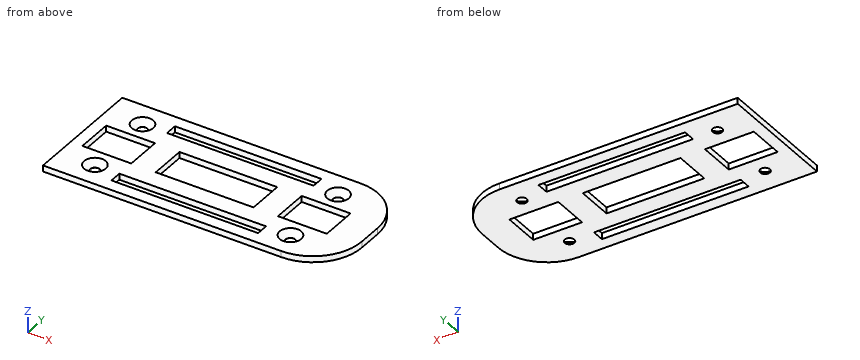
from build123d import *
from build123d import SkipClean  # not in build123d's __all__

# Parameters (mm, degrees)
F1_DEPTH        = 31.75
F1_DEPTH_BACK   = 31.75
F3_R            = 6.35
F4_DEPTH        = 149.1828857926
F5_R            = 12.7
F6_DEPTH        = 25.4
F7_R            = 9.525
F8_DEPTH        = 44.45
F8_DEPTH_BACK   = 66.9427915833
F10_D           = 4.2
F10_DEPTH       = 25.4
F10_TIP         = 1.2618073
F12_DEPTH       = 3.175
F14_D           = 5
F14_CSINK_D     = 11.2
F14_CSINK_ANGLE = 90
F15_W           = 25.4
F15_H           = 19.05
F15_W_2         = 76.2
F15_H_2         = 6.35
F15_W_3         = 50.8
F16_DEPTH       = 41.2760001


# Not quite as in the source:
# - a feature of the source that left no trace in its solid (it failed there, or was rolled back) is left out


with BuildPart() as f1:
    # F0 (on Front) → F1 (new body, two sides)
    with BuildSketch(Plane.XZ) as f1_sk:
        with BuildLine():
            Line((66.9417914833, 19.05), (-82.2400942093, 19.05))
            Line((-82.2400942093, 19.05), (-82.2400942093, -19.05))
            add(Edge.make_bspline(
                [(-82.2400942093, -19.05), (0, -19.05), (66.9417914833, -19.05), (66.9417914833, 19.05)],
                knots=[0, 0, 0, 0, 153.970273166, 153.970273166, 153.970273166, 153.970273166], degree=3))
        make_face()
    extrude(amount=F1_DEPTH)
    extrude(f1_sk.sketch, amount=-F1_DEPTH_BACK)

    # F3 (on face) → F4 (cut, through all)
    with BuildSketch(Plane(origin=(-82.2400942093, 0, 0), x_dir=(0, -1, 0), z_dir=(-1, 0, 0))):
        Circle(F3_R)
    extrude(amount=-F4_DEPTH, mode=Mode.SUBTRACT)

    # F5 (on face) → F6 (cut)
    with BuildSketch(Plane(origin=(-82.2400942093, 0, 0), x_dir=(0, -1, 0), z_dir=(-1, 0, 0))):
        Circle(F5_R)
    extrude(amount=-F6_DEPTH, mode=Mode.SUBTRACT)

    # F7 (on Right) → F8 (cut, two sides)
    with BuildSketch(Plane.YZ) as f8_sk:
        Circle(F7_R)
    extrude(amount=-F8_DEPTH, mode=Mode.SUBTRACT)
    extrude(f8_sk.sketch, amount=F8_DEPTH_BACK, mode=Mode.SUBTRACT)

    # F10
    with Locations(Plane.XY.offset(19.05)):
        with Locations((-63.5, 19.05), (-63.5, -19.05), (25.4, 19.05), (25.4, -19.05)):
            Hole(F10_D / 2, depth=F10_DEPTH)
            with Locations((0, 0, -(F10_DEPTH + F10_TIP / 2))):  # 118° drill point
                Cone(0, F10_D / 2, F10_TIP, mode=Mode.SUBTRACT)


with BuildPart() as f12:
    # F11 (on face) → F12 (new body)
    with BuildSketch(Plane.XY.offset(19.05)):
        with BuildLine():
            Line((41.5417914833, 31.75), (-82.2400942093, 31.75))
            Line((-82.2400942093, 31.75), (-82.2400942093, -31.75))
            Line((-82.2400942093, -31.75), (41.5417914833, -31.75))
            ThreePointArc((41.5417914833, -31.75), (59.5023037254, -24.3105122421), (66.9417914833, -6.35))
            Line((66.9417914833, -6.35), (66.9417914833, 6.35))
            ThreePointArc((66.9417914833, 6.35), (59.5023037254, 24.3105122421), (41.5417914833, 31.75))
        make_face()
    extrude(amount=F12_DEPTH)

    # F14 (through all)
    with Locations(Plane.XY.offset(22.225)):
        with Locations((-63.5, 19.05), (-63.5, -19.05), (38.1, -19.05), (38.1, 19.05)):
            CounterSinkHole(F14_D / 2, F14_CSINK_D / 2, counter_sink_angle=F14_CSINK_ANGLE)


with BuildPart() as f16_tool:
    # F15 (on face) → F16 (new body, through all)
    with BuildSketch(Plane.XY.offset(22.225)):
        with Locations((-63.5, 0)):
            Rectangle(F15_W, F15_H)
        with Locations((38.1, 0)):
            Rectangle(F15_W, F15_H)
        with Locations((-12.7, 22.225)):
            Rectangle(F15_W_2, F15_H_2)
        with Locations((-12.7, -22.225)):
            Rectangle(F15_W_2, F15_H_2)
        with Locations((-12.7, 0)):
            Rectangle(F15_W_3, F15_H)
    extrude(amount=-F16_DEPTH)


with BuildPart() as f1_1:
    add(f1.part, clean=False)

    # F16: cut by f16_tool
    with SkipClean():  # cleaning this boolean's faces spoils the solid; the shape is the same uncleaned
        add(f16_tool.part, mode=Mode.SUBTRACT)


with BuildPart() as f12_1:
    add(f12.part, clean=False)

    # F16: cut by f16_tool
    with SkipClean():  # cleaning this boolean's faces spoils the solid; the shape is the same uncleaned
        add(f16_tool.part, mode=Mode.SUBTRACT)


solid = f12_1.part
Can you work these out from the model? Positions are in its coordinate system, mm. Coordinates: 2 decimals unless noted, no trailing zeros. Write each loop counter-clockwise with the first axis right and the second up, starting at its lowest first coordinate (ties: lowest second). Pieces come first, ordered by that corner, then holes. Notation, with made-up numbers: (-23.75, -33) -> (14.25, -33) arc R7 cw to (14.25, -29) -> close; hole circle Ø3 at (79.5, -15). An arc over 180 degrees is marked (long way). Write each question's results on one line, items separated by ' | '. Start each with the question number.
Item 1: If we section it at B-B, the plane y = -2.5: Write out the boundary of the cut face in (x, z) (3 decimals).
Item 2: I'm going to push flat-ended pins straight in: P1, Ø6, axis at x = 38.1, y = 19.05, coming from the +Z side (3 decimals); P2, Ø1.5, axis at x = -32, y = -19.5, coming from the +Z side (3 decimals). Where does each tip first touch, or does it pass through?
Item 3: If we section it at D-D, the plane x = -63.5: Write out the boundary of the cut face in (y, z) (3 decimals).
Item 4: If we section it at A-A, the plane x = -28: Write out the boundary of the cut face in (y, z) (3 decimals), and give its area (3 significant figures).
Item 5: If we section it at C-C, the plane z = 19.9: Count the separate pieces of the cut face and the enclosed holes in it, and give its area (3 significant figures).
Item 6: Please list where these lines run through material, in increasing order: probe 1 along Y at (x, z) = (-63.5, 19.15) (3 decimals); probe 2 along Y at (x, z) = (-2, 19.55) (3 decimals); probe 3 along X at (y, z) = (-15, 21.7).
Answer block:
1) outline: (-82.24, 19.05) -> (-76.2, 19.05) -> (-76.2, 22.225) -> (-82.24, 22.225) -> close; (-50.8, 19.05) -> (-38.1, 19.05) -> (-38.1, 22.225) -> (-50.8, 22.225) -> close; (12.7, 19.05) -> (25.4, 19.05) -> (25.4, 22.225) -> (12.7, 22.225) -> close; (50.8, 19.05) -> (66.942, 19.05) -> (66.942, 22.225) -> (50.8, 22.225) -> close
2) P1: z = 19.625 | P2: z = 22.225
3) outline: (-31.75, 19.05) -> (-21.55, 19.05) -> (-21.55, 19.125) -> (-24.65, 22.225) -> (-31.75, 22.225) -> close; (-16.55, 19.05) -> (-9.525, 19.05) -> (-9.525, 22.225) -> (-13.45, 22.225) -> (-16.55, 19.125) -> close; (9.525, 19.05) -> (16.55, 19.05) -> (16.55, 19.125) -> (13.45, 22.225) -> (9.525, 22.225) -> close; (21.55, 19.05) -> (31.75, 19.05) -> (31.75, 22.225) -> (24.65, 22.225) -> (21.55, 19.125) -> close
4) outline: (-31.75, 19.05) -> (-25.4, 19.05) -> (-25.4, 22.225) -> (-31.75, 22.225) -> close; (-19.05, 19.05) -> (-9.525, 19.05) -> (-9.525, 22.225) -> (-19.05, 22.225) -> close; (9.525, 19.05) -> (19.05, 19.05) -> (19.05, 22.225) -> (9.525, 22.225) -> close; (25.4, 19.05) -> (31.75, 19.05) -> (31.75, 22.225) -> (25.4, 22.225) -> close | area: 101 mm²
5) separate pieces: 1 | enclosed holes: 9 | area: 6,160 mm²
6) probe 1: -31.75 to -21.575, -16.525 to -9.525, 9.525 to 16.525, 21.575 to 31.75 | probe 2: -31.75 to -25.4, -19.05 to -9.525, 9.525 to 19.05, 25.4 to 31.75 | probe 3: -82.24 to -66.56, -60.44 to 35.04, 41.16 to 65.42
